from build123d import *

# Parameters (mm, degrees)
SKETCH1_W           = 17
SKETCH1_H           = 17
BOSS_EXTRUDE1_DEPTH = 16
CUT_EXTRUDE1_DEPTH  = 29.879058156
CHAMFER1_SIZE       = 1
FILLET1_R           = 2
BOSS_EXTRUDE2_DEPTH = 0.5
CHAMFER3_SIZE       = 1


with BuildPart() as part:
    # Sketch1 → Boss-Extrude1 (new body)
    with BuildSketch(Plane.XY):
        with Locations((8.5, 8.5)):
            Rectangle(SKETCH1_W, SKETCH1_H)
    extrude(amount=BOSS_EXTRUDE1_DEPTH)

    # Sketch2 → Cut-Extrude1 (cut, through all)
    with BuildSketch(Plane.ZY):
        with BuildLine():
            Line((8.953848021, 10.6), (0, 10.6))
            Line((0, 10.6), (0, 6.4))
            Line((0, 6.4), (8.953848021, 6.4))
            ThreePointArc((8.953848021, 6.4), (11.053848021, 8.5), (8.953848021, 10.6))
        make_face()
    extrude(amount=-CUT_EXTRUDE1_DEPTH, mode=Mode.SUBTRACT)

    # Chamfer1
    chamfer1_edges = [part.edges().sort_by_distance(p)[0] for p in [
        (0, 3.2, 0),
        (17, 13.8, 0),
        (17, 8.5, 11.053848021),
        (17, 6.4, 4.47692401),
        (8.5, 6.4, 0),
        (17, 10.6, 4.47692401),
        (8.5, 10.6, 0),
        (0, 8.5, 11.053848021),
        (0, 10.6, 4.47692401),
        (0, 6.4, 4.47692401),
        (8.5, 17, 0),
        (17, 3.2, 0),
        (8.5, 0, 0),
        (0, 13.8, 0),
    ]]
    chamfer(chamfer1_edges, length=CHAMFER1_SIZE)

    # Fillet1
    fillet1_edges = [part.edges().sort_by_distance(p)[0] for p in [
        (8.5, 17, 16),
        (8.5, 0, 16),
    ]]
    fillet(fillet1_edges, radius=FILLET1_R)

    # Sketch3 → Boss-Extrude2 (add)
    with BuildSketch(Plane.XY.offset(16)):
        Polygon((3.244919175, 10.668082206), (4.269558598, 10.668082206), (5.524466451, 6.831744065), (6.788188406, 10.668082206), (7.802911963, 10.668082206), (8.732799784, 5.168082206), (7.733500906, 5.168082206), (7.146261322, 8.641940379), (6.002631515, 5.168082206), (5.039690809, 5.168082206), (3.902671579, 8.641940379), (3.316533758, 5.168082206), (2.316133117, 5.168082206), align=None)
        with BuildLine():
            Line((10.495620297, 9.328338616), (9.508440809, 9.328338616))
            add(Edge.make_bspline(
                [(9.508440809, 9.328338616), (9.515410672, 9.377684197), (9.529074626, 9.47442294), (9.56177064, 9.61447654), (9.600878602, 9.747326965), (9.649702894, 9.872553504), (9.706965845, 9.990379227), (9.772085156, 10.101208455), (9.84576479, 10.204565488), (9.90224101, 10.266828175), (9.93041597, 10.297889898)],
                knots=[0, 0, 0, 0, 1.111473889, 2.178970933, 3.205615836, 4.199322666, 5.174200091, 6.12565194, 7.064921805, 8, 8, 8, 8], degree=3))
            add(Edge.make_bspline(
                [(9.93041597, 10.297889898), (9.971054616, 10.338873592), (10.051149118, 10.419648144), (10.184996423, 10.523111423), (10.325293118, 10.612651854), (10.474852914, 10.683640156), (10.631348547, 10.741096963), (10.796024526, 10.779690829), (10.968207924, 10.805298201), (11.085701432, 10.807820616), (11.145660361, 10.809107847)],
                knots=[0, 0, 0, 0, 1.01925491, 2.00884431, 2.983262333, 3.955970413, 4.92937149, 5.924503185, 6.940838805, 8, 8, 8, 8], degree=3))
            add(Edge.make_bspline(
                [(11.145660361, 10.809107847), (11.198966933, 10.807849383), (11.303756913, 10.805375497), (11.457771816, 10.785516482), (11.604612137, 10.750685982), (11.745830021, 10.705145883), (11.879348613, 10.643180969), (12.008114798, 10.571252892), (12.128530844, 10.483030116), (12.240878502, 10.383347258), (12.344091254, 10.275530489), (12.433473949, 10.160283229), (12.510317856, 10.040683999), (12.573627071, 9.915739156), (12.622303254, 9.785237276), (12.656085968, 9.649932253), (12.678197575, 9.510122647), (12.680400469, 9.415095941), (12.681517733, 9.366900315)],
                knots=[0, 0, 0, 0, 1.091422571, 2.145516843, 3.172569842, 4.178562979, 5.178154469, 6.181868002, 7.194278174, 8.227918432, 9.254613415, 10.245994977, 11.209837596, 12.161663635, 13.10878368, 14.055455738, 15.013766427, 16, 16, 16, 16], degree=3))
            add(Edge.make_bspline(
                [(12.681517733, 9.366900315), (12.679225042, 9.307214046), (12.674711438, 9.189710131), (12.637674052, 9.017734423), (12.579700472, 8.853294955), (12.495951997, 8.698692484), (12.391245073, 8.55434775), (12.262773184, 8.425086631), (12.114195543, 8.308882488), (12.002656329, 8.246434368), (11.945540168, 8.214456405)],
                knots=[0, 0, 0, 0, 0.992805628, 1.954529043, 2.915727527, 3.886831945, 4.871318353, 5.87440735, 6.911542536, 8, 8, 8, 8], degree=3))
            add(Edge.make_bspline(
                [(11.945540168, 8.214456405), (11.984743825, 8.201585019), (12.061777251, 8.176293323), (12.171271003, 8.126481615), (12.275387051, 8.072045674), (12.372332552, 8.00880546), (12.463071747, 7.939318128), (12.547051478, 7.862989674), (12.624773506, 7.77998653), (12.69496905, 7.689852211), (12.757270338, 7.594028239), (12.813169966, 7.494728091), (12.859178476, 7.390445863), (12.898153411, 7.282372527), (12.927826708, 7.169536779), (12.948719361, 7.052375846), (12.960795827, 6.931156981), (12.962637694, 6.849031274), (12.963569015, 6.807505283)],
                knots=[0, 0, 0, 0, 1.059543567, 2.081955587, 3.086750234, 4.076226789, 5.052108497, 6.020845489, 6.989030705, 7.970690546, 8.952259656, 9.923888338, 10.895517021, 11.877585046, 12.873342345, 13.889638361, 14.932918083, 16, 16, 16, 16], degree=3))
            add(Edge.make_bspline(
                [(12.963569015, 6.807505283), (12.961681103, 6.746478937), (12.957958525, 6.626147412), (12.93429212, 6.448911389), (12.890229538, 6.279932588), (12.83226277, 6.117266652), (12.754941393, 5.96301354), (12.663947131, 5.813633354), (12.5520969, 5.674306556), (12.427794574, 5.541349707), (12.289749595, 5.420471294), (12.140086379, 5.315675149), (11.982095893, 5.225741411), (11.814778577, 5.15273064), (11.638192558, 5.096503997), (11.452731433, 5.055860787), (11.257615945, 5.030994598), (11.124434358, 5.02838785), (11.056417572, 5.027056565)],
                knots=[0, 0, 0, 0, 1.005138573, 1.981928558, 2.936866704, 3.876260664, 4.820238198, 5.773547, 6.751179199, 7.756627054, 8.768222608, 9.766606018, 10.760583154, 11.757261445, 12.767156078, 13.807575856, 14.880313354, 16, 16, 16, 16], degree=3))
            add(Edge.make_bspline(
                [(11.056417572, 5.027056565), (10.99207479, 5.02846018), (10.866260993, 5.031204763), (10.682231983, 5.054960522), (10.507329828, 5.093280489), (10.341108177, 5.147295661), (10.184210125, 5.217344107), (10.035212862, 5.300756089), (9.897089595, 5.402342616), (9.768301357, 5.517517881), (9.651705062, 5.646737988), (9.547495432, 5.787009618), (9.457970308, 5.938866167), (9.382762546, 6.10165884), (9.3224601, 6.275673225), (9.274893708, 6.460555454), (9.241667805, 6.656666729), (9.231548786, 6.791595459), (9.226389527, 6.860389898)],
                knots=[0, 0, 0, 0, 1.066544725, 2.085487077, 3.070979577, 4.031932826, 4.977951092, 5.916076795, 6.857635327, 7.814973522, 8.776389752, 9.738577119, 10.707772778, 11.69409279, 12.707140348, 13.757286496, 14.856535458, 16, 16, 16, 16], degree=3))
            Line((9.226389527, 6.860389898), (10.213569015, 6.860389898))
            add(Edge.make_bspline(
                [(10.213569015, 6.860389898), (10.219824668, 6.825799151), (10.232009194, 6.7584246), (10.255774364, 6.660881227), (10.286743696, 6.570842669), (10.322551949, 6.487508666), (10.361230253, 6.409785071), (10.407962894, 6.340542409), (10.459325549, 6.277900458), (10.533442235, 6.203431016), (10.639397142, 6.126916773), (10.782471369, 6.060422256), (10.941627897, 6.0214483), (11.052894184, 6.016693597), (11.110403951, 6.014236052)],
                knots=[0, 0, 0, 0, 0.928156231, 1.807827665, 2.648129825, 3.438902246, 4.202261636, 4.936546065, 5.639352463, 6.338805438, 7.70633318, 9.064371875, 10.482673459, 12, 12, 12, 12], degree=3))
            add(Edge.make_bspline(
                [(11.110403951, 6.014236052), (11.140920666, 6.014759363), (11.200696083, 6.015784412), (11.288497271, 6.027145709), (11.372140265, 6.045857774), (11.451780855, 6.071286777), (11.527926037, 6.103163621), (11.599120982, 6.144266905), (11.66681682, 6.192055339), (11.730277635, 6.245782226), (11.788916737, 6.304325301), (11.837707918, 6.369151809), (11.882299527, 6.435027129), (11.915279803, 6.506261054), (11.944177629, 6.57902044), (11.961864575, 6.655946223), (11.975219489, 6.735424708), (11.975995623, 6.789816294), (11.976389527, 6.817421148)],
                knots=[0, 0, 0, 0, 1.110435564, 2.175094844, 3.216326037, 4.226890168, 5.215276772, 6.21526065, 7.213097102, 8.228249917, 9.239874822, 10.221364777, 11.178138315, 12.128914389, 13.072518965, 14.022636769, 14.996447288, 16, 16, 16, 16], degree=3))
            add(Edge.make_bspline(
                [(11.976389527, 6.817421148), (11.975343786, 6.84761176), (11.973261954, 6.907714349), (11.95625317, 6.99542144), (11.929392706, 7.079788593), (11.892080239, 7.16044219), (11.842253599, 7.237084958), (11.783458719, 7.311254584), (11.711063536, 7.37909067), (11.631636324, 7.446144585), (11.539531961, 7.504595376), (11.43923606, 7.558536867), (11.328112687, 7.601457641), (11.208874464, 7.639793843), (11.079265887, 7.667794008), (10.94009178, 7.688124858), (10.791576649, 7.703258025), (10.689203239, 7.705429126), (10.636645938, 7.706543745)],
                knots=[0, 0, 0, 0, 0.809814727, 1.612155564, 2.388397, 3.182215007, 3.988903953, 4.837162975, 5.715530372, 6.646997145, 7.623086902, 8.637258368, 9.698941581, 10.815059213, 11.996518529, 13.252603015, 14.589518788, 16, 16, 16, 16], degree=3))
            Line((10.636645938, 7.706543745), (10.636645938, 8.623210411))
            add(Edge.make_bspline(
                [(10.636645938, 8.623210411), (10.702082904, 8.628783233), (10.824502508, 8.639208878), (10.994427483, 8.663589612), (11.137482407, 8.696178476), (11.257105609, 8.735495178), (11.356433051, 8.785988065), (11.443204956, 8.841729984), (11.517937025, 8.906466075), (11.581095648, 8.978265919), (11.631620581, 9.055372218), (11.667379186, 9.136586513), (11.6909923, 9.219395932), (11.693229641, 9.276035079), (11.694338245, 9.304099834)],
                knots=[0, 0, 0, 0, 1.70044513, 3.18119609, 4.440695891, 5.496282586, 6.431922213, 7.318171381, 8.16090191, 8.983045123, 9.787564368, 10.536848927, 11.275007137, 12, 12, 12, 12], degree=3))
            add(Edge.make_bspline(
                [(11.694338245, 9.304099834), (11.692425585, 9.339907415), (11.688692477, 9.409796232), (11.659699137, 9.509821852), (11.609369984, 9.598986402), (11.541887427, 9.677102254), (11.459657586, 9.742350468), (11.363269796, 9.789719559), (11.254815679, 9.817551015), (11.178512364, 9.820436199), (11.139049784, 9.82192836)],
                knots=[0, 0, 0, 0, 1.009664648, 1.970651636, 2.907870547, 3.878035693, 4.867062054, 5.849714035, 6.887914197, 8, 8, 8, 8], degree=3))
            add(Edge.make_bspline(
                [(11.139049784, 9.82192836), (11.103281391, 9.820167767), (11.032305946, 9.816674212), (10.9285186, 9.79059924), (10.8299552, 9.746705269), (10.738656716, 9.686178071), (10.655941059, 9.613487472), (10.588055369, 9.527400545), (10.531591271, 9.433074908), (10.507657627, 9.363387579), (10.495620297, 9.328338616)],
                knots=[0, 0, 0, 0, 0.98818071, 1.960853194, 2.938124878, 3.957524365, 4.978590984, 5.968022688, 6.978025184, 8, 8, 8, 8], degree=3))
        make_face()
    extrude(amount=BOSS_EXTRUDE2_DEPTH)

    # Chamfer3
    chamfer3_edges = [part.edges().sort_by_distance(p)[0] for p in [
        (0, 8.5, 16),
        (17, 8.5, 16),
        (17, 0, 7.5),
        (17, 17, 7.5),
        (17, 16.414213562, 15.414213562),
        (17, 0.585786438, 15.414213562),
        (0, 0, 7.5),
        (0, 17, 7.5),
        (0, 16.414213562, 15.414213562),
        (0, 0.585786438, 15.414213562),
    ]]
    chamfer(chamfer3_edges, length=CHAMFER3_SIZE)


solid = part.part
Build history of the part. All positions in model axes, mm. A direction names the side the tool comes from. Coordinates: 2 decimals unless noted, no trailing zeros. Order: outer loops, then holes, each group sorted by start corner. A loop starts at its lowest first (then second) coordinate and runs counter-clockwise, first axis right, second up. Notation, with made-up numbers: M -30,11 L 9,11 A25 ccw 9,48 Z; hole C 46,83 d1. An arc over 180 degrees is marked long. One line per question, with ' | ' between items. Start each with the question number.
Q1. Saw through at A-A (z = 2.75). List the corners of the cut face in (x, y).
Q2. Flat gauge pins, fed straight in: pin 1 Ø4 at (x, y) = (12, 9) entering from -Z; pin 2 Ø0.6 at (x, z) = (5.5, 16) entering from -Y. Where does each tip first touch, or does it go through?
Q3. 3-axis set-ups, long thin cutter, end or side, ignore diameter. For faces 1 (the face through (4.888, 8.777, 16.247)), 2 (the face through (8.4, 5.9, 0.5)), 3 (the face through (0.5, 11.1, 5)), 4 (the face through (8, 17, 7)), 5 (the face through (16.3, 5.7, 0.6)): which of +Z, -Z, +X, -X, +Y, -Y reach the whole face in a straight line?
Q4. Saw through at C-C (y = 3). List the corners of the cut face in (x, z).
Q5. Probe L1, parallel to Y at x = 13.75, z = 4.5; L2, parallel to Z at x = 13, y = 14.5; L3, parallel to Y at x = 14.75, z = 0.5. List the from-to ranges inside material, lowest first. Write a range as from..to.
Q6. Saw through at B-B (x = 2). List the corners of the cut face in (y, z), then the cut area to 3 significant figures.
Q7. Two-plate mould, pull along X, no slides. Class faces 6 (the face through (4.48, 6.88, 16.25)), 7 (the face through (0.5, 14, 0.5)), 8 (the face through (16.5, 5.9, 4.9)), 9 (the face through (8.26, 7.96, 16.25)): +X half, -X half, draft (parallel to the pull), parting line (faces both ways), or undercut.
Check values:
1) outline: M 0,1 L 1,0 L 16,0 L 17,1 L 17,5.4 L 16,6.4 L 1,6.4 L 0,5.4 Z; M 0,11.6 L 1,10.6 L 16,10.6 L 17,11.6 L 17,16 L 16,17 L 1,17 L 0,16 Z
2) pin 1: stops at z = 0.6 | pin 2: stops at y = 0.95
3) face 1: +Z, +Y | face 2: -Z, +X, -X | face 3: -Z, -X | face 4: +Z, -Z, +X, -X, +Y | face 5: -Z, +X
4) outline: M 0,1 L 1,0 L 16,0 L 17,1 L 17,15 L 16,16 L 1,16 L 0,15 Z
5) L1: y = 0..6.4, 10.6..17 | L2: z = 0..16 | L3: y = 0.5..5.9, 11.1..16.5
6) outline: M 0,1 L 1,0 L 5.4,0 L 6.4,1 L 6.4,8.95 A2.1 cw 10.6,8.95 L 10.6,1 L 11.6,0 L 16,0 L 17,1 L 17,14 A2 ccw 15,16 L 2,16 A2 ccw 0,14 Z | area: 224 mm2
7) face 6: undercut | face 7: -X half | face 8: +X half | face 9: undercut
